from build123d import *

# Parameters (mm, degrees)
F1_DEPTH = 2.032


with BuildPart() as f1:
    # F0 (on Top) → F1 (new body)
    with BuildSketch(Plane.XY):
        Polygon((59.5508336694, 40.6870045497), (34.1508336694, 40.6870045497), (4.7581588602, 101.8170116116), (-24.634515949, 40.6870045497), (-50.034515949, 40.6870045497), (-67.0533862158, 5.2916665496), (-72.6509597748, -6.3499997298), (-65.0918408696, -6.3499997298), (-65.0918408696, -57.1499997298), (74.60815859, -57.1499997298), (74.60815859, -6.3499997298), (82.1672774952, -6.3499997298), (76.5697039363, 5.2916665496), align=None)
        Polygon((4.7581588602, 91.852396227), (31.4358146836, 36.3690045497), (56.8358146836, 36.3690045497), (72.6781767233, 3.4205332163), (75.2998765312, -2.0319997298), (70.29015859, -2.0319997298), (70.29015859, -52.8319997298), (-60.7738408696, -52.8319997298), (-60.7738408696, -2.0319997298), (-65.7835588108, -2.0319997298), (-63.1618590029, 3.4205332163), (-47.3194969632, 36.3690045497), (-23.4601999485, 36.3690045497), (-21.9194969632, 36.3690045497), align=None, mode=Mode.SUBTRACT)
        Polygon((56.8358146836, 36.3690045497), (31.4358146836, 36.3690045497), (4.7581588602, 91.852396227), (-21.9194969632, 36.3690045497), (-23.4601999485, 36.3690045497), (-47.3194969632, 36.3690045497), (-63.1618590029, 3.4205332163), (-65.7835588108, -2.0319997298), (-60.7738408696, -2.0319997298), (-60.7738408696, -52.8319997298), (70.29015859, -52.8319997298), (70.29015859, -2.0319997298), (75.2998765312, -2.0319997298), (72.6781767233, 3.4205332163), align=None)
        Polygon((68.2581588602, -50.8), (-58.7418411398, -50.8), (-58.7418411398, 0), (-62.5518411398, 0), (-61.8190678495, 1.524), (-46.0418411398, 34.3370048199), (-22.332856425, 34.3370048199), (-20.6418411398, 34.3370048199), (-18.376729311, 39.0479167388), (-8.5820728345, 59.4185506966), (-5.3240396144, 66.1945108652), (4.7581588602, 87.1631660812), (14.8403573348, 66.1945108652), (18.0983905549, 59.4185506966), (27.8930470314, 39.0479167388), (30.1581588602, 34.3370048199), (31.8491741455, 34.3370048199), (55.5581588602, 34.3370048199), (71.3353855699, 1.524), (72.0681588602, 0), (68.2581588602, 0), align=None, mode=Mode.SUBTRACT)
    extrude(amount=-F1_DEPTH)


solid = f1.part
Design review of the part built by this model. Coordinates are the model's own, in mm. Coordinates: 2 decimals unless noted, no trailing zeros. Loops run counter-clockwise (first coordinate to the right, second up) from the corner with the lowest first, then second, coordinate; pieces in that order, holes last. Notation, with made-up numbers: M -4,-28.5 L 22,-28.5 A36 cw 22,8.5 Z; hole C 82.25,84.5 d7. An arc over 180 degrees is marked long. Use one line per item in the form item = value.
(1) For line 1 along Y through (x, z) = (36, -1.45); line 2 along X through (y, z) = (-21.5, -1.15); line 3 along Y through (x, z) = (57, -1.5), list the stretches that pass through material, from the lowest coordinate up. Write a range as from..to.
Return value:
line_1 = -57.15..-50.8, 34.34..40.69
line_2 = -65.09..-58.74, 68.26..74.61
line_3 = -57.15..-50.8, 31.34..40.69
(2) Consider section A-A (y = -11). Write out the cut boundary in (x, z), and give its area (3 significant figures).
Return value:
outline = M -65.09,-2.03 L -58.74,-2.03 L -58.74,0 L -65.09,0 Z; M 68.26,-2.03 L 74.61,-2.03 L 74.61,0 L 68.26,0 Z
area = 25.8 mm2
(3) Consider section C-C (z = -1.45). Write out the cut boundary in (x, y).
Return value:
outline = M -72.65,-6.35 L -65.09,-6.35 L -65.09,-57.15 L 74.61,-57.15 L 74.61,-6.35 L 82.17,-6.35 L 59.55,40.69 L 34.15,40.69 L 4.76,101.82 L -24.63,40.69 L -50.03,40.69 Z; hole M -62.55,0 L -58.74,0 L -58.74,-50.8 L 68.26,-50.8 L 68.26,0 L 72.07,0 L 55.56,34.34 L 30.16,34.34 L 4.76,87.16 L -20.64,34.34 L -46.04,34.34 Z
(4) Consider section B-B (x = 46.5). Write out the cut boundary in (y, z).
Return value:
outline = M -57.15,-2.03 L -50.8,-2.03 L -50.8,0 L -57.15,0 Z; M 34.34,-2.03 L 40.69,-2.03 L 40.69,0 L 34.34,0 Z
(5) Draft analysis for pull direction X (two halves, no side actions). For faces 1 (the face through (-9.732, 71.68, -1.002)), 2 (the face through (19.66, 70.82, -1)), 3 (the face through (33.1, 34.5, 0)), state which applies: pulls with the +X half, pulls with the -X half, needs draft (parallel to the pull), parting line crosses it, or undercut.
Return value:
face_1 = pulls with the -X half
face_2 = pulls with the +X half
face_3 = needs draft
(6) Clearance check with flat-ended pins moving along their axes: P1, Ø1, axis at x = 41, z = -1.5, coming from the +Y side; P2, Ø0.6, axis at x = 70.5, z = -1.5, coming from the +Y side; P3, Ø0.6, axis at x = -70.5, z = -0.5, coming from the -Y side. State where each tip first meets the part, or that it passes through.
Return value:
P1 = 40.69
P2 = 18.54
P3 = -6.35
